```python
from build123d import *

# Parameters (mm, degrees)
SKETCH_R  = 1.7
PAD_DEPTH = 1.5


with BuildPart() as part:
    # Sketch → Pad (new body)
    with BuildSketch(Plane.XY):
        Polygon((-27.5, 19), (27.5, 19), (27.5, -19), (10, -19), (10, -2), (-10, -2), (-10, -19), (-27.5, -19), align=None)
        with Locations((-8, 2.85)):
            Circle(SKETCH_R, mode=Mode.SUBTRACT)
        with Locations((8, 2.85)):
            Circle(SKETCH_R, mode=Mode.SUBTRACT)
        with BuildLine():
            ThreePointArc((-10, 17.5), (-13, 14.5), (-10, 11.5))
            Line((-10, 11.5), (10, 11.5))
            ThreePointArc((10, 11.5), (13, 14.5), (10, 17.5))
            Line((-10, 17.5), (10, 17.5))
        make_face(mode=Mode.SUBTRACT)
        with BuildLine():
            ThreePointArc((23.485, 5.38), (20.485, 8.38), (17.485, 5.38))
            Line((17.485, 5.38), (17.485, -14.62))
            ThreePointArc((17.485, -14.62), (20.485, -17.62), (23.485, -14.62))
            Line((23.485, 5.38), (23.485, -14.62))
        make_face(mode=Mode.SUBTRACT)
        with BuildLine():
            ThreePointArc((-23.485, -14.62), (-20.485, -17.62), (-17.485, -14.62))
            Line((-17.485, -14.62), (-17.485, 5.38))
            ThreePointArc((-17.485, 5.38), (-20.485, 8.38), (-23.485, 5.38))
            Line((-23.485, -14.62), (-23.485, 5.38))
        make_face(mode=Mode.SUBTRACT)
    extrude(amount=PAD_DEPTH)


solid = part.part
```
Build history of the part. All positions in model axes, mm. A direction names the side the tool comes from. Give positions to 0.01 mm unless a question says otherwise; leave off trailing zeros. Order: outer loops, then holes, each group sorted by start corner. A loop starts at its lowest first (then second) coordinate and runs counter-clockwise, first axis right, second up. Notation, with made-up numbers: M 13,20.5 L 27,20.5 A16 ccw 27,44.5 Z; hole C 89.25,34.5 d3. An arc over 180 degrees is marked long. Return JSON: item names as keys, results as strings.
Q1. Wall check: probe 1 along X at (y, z) = (-7, 1.3) (3 decimals); probe 2 along Y at (x, z) = (8, 0.4); probe 3 along Y at (x, z) = (-20.5, 1). Give the ranges that are in metal, low to high. Write a range as from..to.
Answer list:
{"probe 1": "x = -27.5..-23.485, -17.485..-10, 10..17.485, 23.485..27.5", "probe 2": "y = -2..1.15, 4.55..11.5, 17.5..19", "probe 3": "y = -19..-17.62, 8.38..19"}
Q2. Band-saw the part on A-A (y = 14.5). Give the cut face in (x, z), then the cut area to 3 significant figures.
Answer list:
{"outline": "M -27.5,0 L -13,0 L -13,1.5 L -27.5,1.5 Z; M 13,0 L 27.5,0 L 27.5,1.5 L 13,1.5 Z", "area": "43.5 mm^2"}
Q3. Band-saw the part on D-D (y = -3). Give the cut face in (x, z) (3 decimals), then the cut area to 3 significant figures.
Answer list:
{"outline": "M -27.5,0 L -23.485,0 L -23.485,1.5 L -27.5,1.5 Z; M -17.485,0 L -10,0 L -10,1.5 L -17.485,1.5 Z; M 10,0 L 17.485,0 L 17.485,1.5 L 10,1.5 Z; M 23.485,0 L 27.5,0 L 27.5,1.5 L 23.485,1.5 Z", "area": "34.5 mm^2"}
Q4. 3-axis set-ups, long thin cutter, end or side, ignore diameter. For faces 4 (the face through (0, -2, 1)), 5 (the face through (20.42, -17.62, 0.74)), 6 (the face through (27.5, 0, 1)): which of +Z, -Z, +X, -X, +Y, -Y reach the whole face in a straight line?
Answer list:
{"face 4": "+Z, -Z, -Y", "face 5": "+Z, -Z", "face 6": "+Z, -Z, +X, +Y, -Y"}
Q5. Band-saw the part on C-C (z = 1). Give the cut face in (x, y) (3 decimals).
Answer list:
{"outline": "M -27.5,-19 L -10,-19 L -10,-2 L 10,-2 L 10,-19 L 27.5,-19 L 27.5,19 L -27.5,19 Z; hole M -23.485,-14.62 A3 ccw -17.485,-14.62 L -17.485,5.38 A3 ccw -23.485,5.38 Z; hole M -10,11.5 L 10,11.5 A3 ccw 10,17.5 L -10,17.5 A3 ccw Z; hole C -8,2.85 d3.4; hole C 8,2.85 d3.4; hole M 17.485,-14.62 A3 ccw 23.485,-14.62 L 23.485,5.38 A3 ccw 17.485,5.38 Z"}
Q6. Two-plate mould, pull along X, no slides. Class faces 1 (the face through (13, 14.4, 0.7)), 2 (the face through (-27.5, 0, 1)), 3 (the face through (0, 19, 1)): pulls with the +X half, pulls with the -X half, needs draft (parallel to the pull), parting line crosses it, or undercut.
Answer list:
{"face 1": "undercut", "face 2": "pulls with the -X half", "face 3": "needs draft"}
Q7. Band-saw the part on B-B (x = -5.5). Give the cut face in (y, z).
Answer list:
{"outline": "M -2,0 L 11.5,0 L 11.5,1.5 L -2,1.5 Z; M 17.5,0 L 19,0 L 19,1.5 L 17.5,1.5 Z"}
Q8. Flat gauge pins, fed straight in: pin 1 (2 mm diameter, centred on x = 22, y = 9.5, fed in from -Z); pin 2 (2.5 mm diameter, centred on x = 8, y = 2.85, fed in from +Z); pin 3 (0.8 mm diameter, centred on x = 0.5, z = 0.5, fed in from -Y). Where does each tip first touch, or does it go through?
Answer list:
{"pin 1": "stops at z = 0", "pin 2": "passes through", "pin 3": "stops at y = -2"}
